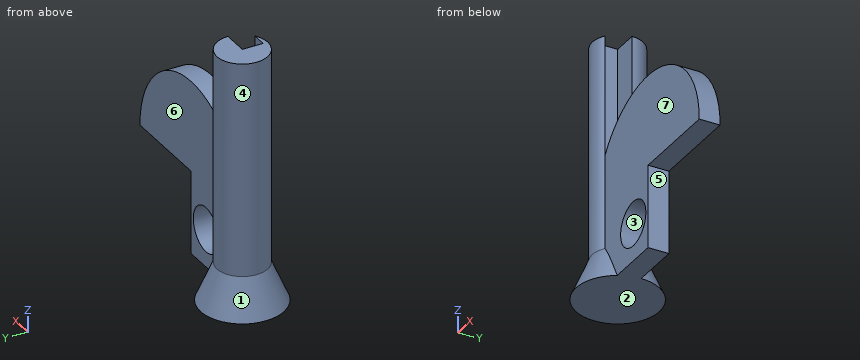
```python
from build123d import *

# Parameters (mm, degrees)
F0_W     = 110.7262298465
F0_H     = 101.6
F0_R     = 27.2882199073
F1_DEPTH = 25.4
F4_DEPTH = 262.128
F5_ANGLE = 180


with BuildPart() as f1:
    # F0 (on Front) → F1 (new body)
    with BuildSketch(Plane.XZ):
        with Locations((55.3631149232, 50.8)):
            Rectangle(F0_W, F0_H)
        with Locations((78.689802438, 45.9539219737)):
            Circle(F0_R, mode=Mode.SUBTRACT)
    extrude(amount=F1_DEPTH)

    # F2 (on Front) → F3 (revolve)
    with BuildSketch(Plane.XZ):
        Polygon((-50.8, 0), (0, 0), (0, 46.7330427111), (-30.9378135865, 46.7330427111), align=None)
    revolve(axis=Axis((0, 0, 23.3665213556), (0, 0, -1)))

    # F4 (add): a face of the model
    f4_faces = [f1.faces().sort_by_distance(p)[0] for p in [
        (-4.0593514792, 3.4603008855, 46.7330427111),
    ]]
    extrude(f4_faces, amount=F4_DEPTH)

    # F1_face (on face) → F5 (revolve)
    with BuildSketch(Plane(origin=(55.3631149232, -12.7, 101.6), x_dir=(1, 0, 0), z_dir=(0, 0, 1))):
        Polygon((55.3631149232, -12.7), (55.3631149232, 12.7), (-24.4253013368, 12.7), (-55.3631149232, 12.7), (-55.3631149232, -12.7), (-37.6999241155, -12.7), align=None)
    revolve(axis=Axis((110.7262298465, -12.7, 101.6), (0, 1, 0)), revolution_arc=F5_ANGLE)


solid = f1.part
```
Can you work these out from the model? Positions are in its coordinate system, mm. Face numbers are marked on the shaded views. A direction names the side the tool comes from. Round coordinates to 2 decimals unless told otherwise and drop trailing zeros. Loops run counter-clockwise (first coordinate to the right, second up) from the corner with the lowest first, then second, coordinate; pieces in that order, holes last. Notation, with made-up numbers: M -17,73 L -11,73 A27 cw -11,89 Z; hole C 38.5,-14.5 d7. An arc over 180 degrees is marked long. Write item = value, one per line. Start each with the question number.
(1) Suppose I cut it at C-C on z = 278.5. Write out the boundary of the cut face in (x, y).
(2) If we mould it in two halves opening along Z, with no side actions, what happens to the marked faces 1, 2, 3 and 4? For each: released by +Z, released by -Z, zero draft, split by the parting line, or undercut.
(3) Suppose I cut it at B-B on x = 97.5. Write out the boundary of the cut face in (y, z), plus the area to 3 significant figures.
(4) Which directions (+Z, -Z, +X, -X, +Y, -Y) give clear straight access to the entire face, cutting with the end or side of a thin tool? Please do the marked faces 5, 6 and 7.
(5) Suppose I cut it at A-A on z = 196.5. Write out the boundary of the cut face in (x, y), plus the area to 3 significant figures.
(6) Suppose I cut it at D-D on x = 133.5. Write out the boundary of the cut face in (y, z), plus the area to 3 significant figures.
(7) I need wall thicknesses on line 1 along X through (y, z) = (-2.5, 128); line 2 along Y through (x, z) = (109.5, 203); line 3 along Y through (x, z) = (8, 172.5). Which ranges of each line are inside material? Lowest first, please.
(8) I'm going to push flat-ended pins straight in: P1, Ø20.5, axis at y = -14, z = 179, coming from the +X side; P2, Ø12, axis at x = 9.5, z = 113, coming from the -Y side; P3, Ø6, axis at y = 7, z = 246, coming from the -X side. Where does each tip first touch, or does it pass through?
Answer block:
q1.outline = M 0,-25.4 L 0,0 L 30.94,0 A30.94 ccw long 17.66,-25.4 Z
q2.face_1 = released by +Z
q2.face_2 = released by -Z
q2.face_3 = undercut
q2.face_4 = zero draft
q3.outline = M -25.4,0 L 0,0 L 0,26.18 L -25.4,26.18 Z; M -25.4,65.72 L 0,65.72 L 0,211.53 L -25.4,211.53 Z
q3.area = 4,370 mm²
q4.face_5 = -Z, +X, +Y, -Y
q4.face_6 = +Z, +X, +Y
q4.face_7 = +Z, +X, -Y
q5.outline = M 0,-25.4 L 0,0 L 30.94,0 A30.94 ccw long 17.66,-25.4 Z; M 53.68,-25.4 L 167.77,-25.4 L 167.77,0 L 53.68,0 Z
q5.area = 5,220 mm²
q6.outline = M -25.4,101.6 L 0,101.6 L 0,209.96 L -25.4,209.96 Z
q6.area = 2,750 mm²
q7.line_1 = -30.84 to 0, 3.19 to 218.26
q7.line_2 = -25.4 to 0
q7.line_3 = -29.89 to -25.4, 0 to 29.89
q8.P1 = 198.77
q8.P2 = -30.74
q8.P3 = -30.68
